For this review, take the finished solid that the model builds, in its own axes (mm). Face numbers are marked on the shaded views. A direction names the side the tool comes from. Coordinates: 2 decimals unless noted, no trailing zeros. Loops run counter-clockwise (first coordinate to the right, second up) from the corner with the lowest first, then second, coordinate; pieces in that order, holes last. Notation, with made-up numbers: M 32,62.25 L 66,62.25 A37 cw 66,100.25 Z; hole C 84,-33 d1. An arc over 180 degrees is marked long. Write item = value, one per line.
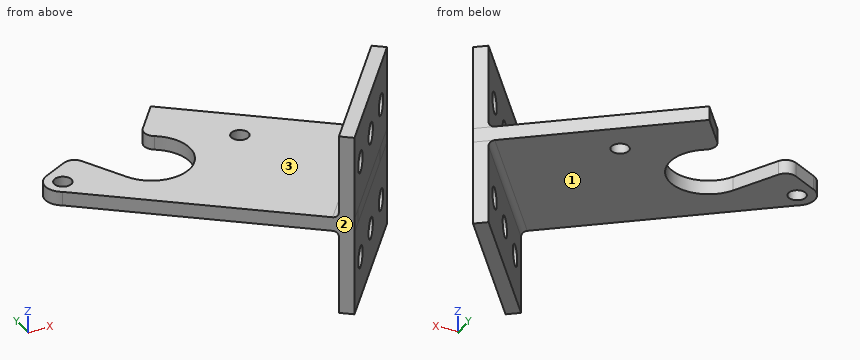
from build123d import *

# Parameters (mm, degrees)
SKETCH1_R           = 3.937
BOSS_EXTRUDE1_DEPTH = 6.35
SKETCH2_W           = 38.1
SKETCH2_H           = 72.406172823
SKETCH2_R           = 4.7625
BOSS_EXTRUDE2_DEPTH = 6.35
FILLET1_R           = 2.54
FILLET2_R           = 5.08


with BuildPart() as part:
    # Sketch1 → Boss-Extrude1 (new body)
    with BuildSketch(Plane.XY):
        with BuildLine():
            ThreePointArc((-16.827513409, -7.862086917), (12.639466563, -9.959944911), (2.148977793, 17.656238065))
            Line((2.148977793, 17.656238065), (16.995641365, 36.92542525))
            Line((16.995641365, 36.92542525), (93.470395294, -21.997399694))
            Line((93.470395294, -21.997399694), (83.897723102, -34.421579135))
            Line((83.897723102, -34.421579135), (54.096930983, -73.099430143))
            Line((54.096930983, -73.099430143), (49.278309192, -79.35342282))
            Line((49.278309192, -79.35342282), (-45.219558371, -6.544018121))
            ThreePointArc((-45.219558371, -6.544018121), (-49.424138371, 0.498338517), (-45.219558371, 7.540695156))
            Line((-45.219558371, 7.540695156), (-29.721187426, 15.893414291))
            Line((-29.721187426, 15.893414291), (-16.827513409, -7.862086917))
        make_face()
        with Locations((-41.424138371, 0.498338517)):
            Circle(SKETCH1_R, mode=Mode.SUBTRACT)
        with Locations((38.575861629, 0.498338517)):
            Circle(SKETCH1_R, mode=Mode.SUBTRACT)
    extrude(amount=BOSS_EXTRUDE1_DEPTH)

    # Sketch2 → Boss-Extrude2 (add)
    # profile 1 of 2: a face of its own
    with BuildSketch(Plane(origin=(69.2868994, -53.384674478, 0), x_dir=(0, 0, -1), z_dir=(0.7921427260999971, -0.6103358923468823, 0))):
        with Locations((19.05, 3.420170547)):
            Rectangle(SKETCH2_W, SKETCH2_H)
        with Locations(Location((19.05, 26.280170547, 0), (0, 0, 90))):
            Circle(SKETCH2_R, mode=Mode.SUBTRACT)
        with Locations(Location((19.05, -19.439829453, 0), (0, 0, 90))):
            Circle(SKETCH2_R, mode=Mode.SUBTRACT)
        with Locations(Location((19.05, 3.420170547, 0), (0, 0, 90))):
            Circle(SKETCH2_R, mode=Mode.SUBTRACT)
    # profile 2 of 2: a face of its own
    with BuildSketch(Plane(origin=(69.2868994, -53.384674478, 0), x_dir=(0, 0, -1), z_dir=(0.7921427260999971, -0.6103358923468823, 0))):
        with Locations((-25.4, 3.420170547)):
            Rectangle(SKETCH2_W, SKETCH2_H)
        with Locations(Location((-25.4, -19.439829453, 0), (0, 0, 90))):
            Circle(SKETCH2_R, mode=Mode.SUBTRACT)
        with Locations(Location((-25.4, 26.280170547, 0), (0, 0, 90))):
            Circle(SKETCH2_R, mode=Mode.SUBTRACT)
        with Locations(Location((-25.4, 3.420170547, 0), (0, 0, 90))):
            Circle(SKETCH2_R, mode=Mode.SUBTRACT)
    extrude(amount=-BOSS_EXTRUDE2_DEPTH)

    # Fillet1
    fillet1_edges = [part.edges().sort_by_distance(p)[0] for p in [
        (66.344245932, -46.799778341, 0),
        (66.344245932, -46.799778341, 6.35),
    ]]
    fillet(fillet1_edges, radius=FILLET1_R)

    # Fillet2
    fillet2_edges = [part.edges().sort_by_distance(p)[0] for p in [
        (2.148977793, 17.656238065, 3.175),
        (-29.721187426, 15.893414291, 3.175),
    ]]
    fillet(fillet2_edges, radius=FILLET2_R)


solid = part.part
Q1. Add section A-A (x = -41). Write out the cut boundary in (y, z), and give its area (3 significant figures).
Solved:
outline = M -9.8,0 L -3.42,0 L -3.42,6.35 L -9.8,6.35 Z; M 4.41,0 L 9.81,0 L 9.81,6.35 L 4.41,6.35 Z
area = 74.8 mm²
Q2. Add section B-B (z = 3.5). Write out the cut boundary in (x, y).
Solved:
outline = M -45.22,-6.54 L 49.28,-79.35 L 93.47,-22 L 17,36.93 L 6.23,22.95 A5.08 ccw 7.63,15.5 A17.53 cw long -16.83,-7.86 L -27.31,11.44 A5.08 ccw -34.18,13.49 L -45.22,7.54 A8 ccw Z; hole C -41.42,0.5 d7.87; hole C 38.58,0.5 d7.87
Q3. Machinability: for the marked faces 1, 2 and 3, which of the approach directions +Z, -Z, +X, -X, +Y, -Y give a long, thin tool a straight path to every point of the face, cutting with its end or side? Answer none if there is none.
Solved:
face_1 = -Z, -X, +Y
face_2 = +Z, -Z, -X, -Y
face_3 = +Z, -X, +Y
Q4. Add section C-C (x = 40). Write out the cut boundary in (y, z).
Solved:
outline = M -72.2,0 L -3.17,0 L -3.17,6.35 L -72.2,6.35 Z; M 4.17,0 L 19.2,0 L 19.2,6.35 L 4.17,6.35 Z
Q5. Add section D-D (y = -67). State how many separate pieces and enclosed holes the cut face has, and give its area (3 significant figures).
Solved:
separate_pieces = 3
enclosed_holes = 0
area = 631 mm²
Q6. For line 1 along Z through (x, y) = (-24.5, -21); line 2 along X through (y, z) = (-41.5, 33), list the stretches that pass through material, from the lowest coordinate up.
Solved:
line_1 = 0 to 6.35
line_2 = 70.43 to 78.44
Q7. For pin 1 Ø10 at (x, z) = (41.5, 14.5) entering from -Y; pin 2 Ø5 at (x, z) = (76.5, -17) entering from +Y; pin 3 Ø4.5 at (x, y) = (-41.42, 0.5) entering from -Z; pin 4 Ø1 at (y, z) = (-18, 21.5) entering from -X, all flat-tipped, find the tip position at first contact; note any pin that passes through.
Solved:
pin_1 = -77.21
pin_2 = -31.12
pin_3 = through
pin_4 = 88.15
